The model under review builds one solid part; all positions refer to its coordinate system, in mm. Coordinates: 2 decimals unless noted, no trailing zeros. Order: outer loops, then holes, each group sorted by start corner. A loop starts at its lowest first (then second) coordinate and runs counter-clockwise, first axis right, second up. Notation, with made-up numbers: M -9,-9.75 L 16,-9.75 A17 ccw 16,4.25 Z; hole C 10.25,71 d3. An arc over 180 degrees is marked long. Answer in a Markdown table with one row per item.
from build123d import *

# Parameters (mm, degrees)
F1_DEPTH = 0.127


with BuildPart() as f1:
    # F0 (on Top) → F1 (new body)
    with BuildSketch(Plane.XY):
        with BuildLine():
            ThreePointArc((0, 1.27), (0.371974, 0.371974), (1.27, 0))
            Line((1.27, 0), (24.13, 0))
            ThreePointArc((24.13, 0), (25.028026, 0.371974), (25.4, 1.27))
            Line((25.4, 1.27), (25.4, 5.08))
            ThreePointArc((25.4, 5.08), (25.028026, 5.978026), (24.13, 6.35))
            Line((24.13, 6.35), (16.191119, 6.35))
            ThreePointArc((16.191119, 6.35), (15.720802, 6.234588), (15.357337, 5.914571))
            ThreePointArc((15.357337, 5.914571), (14.503814, 5.622968), (13.97, 6.35))
            Line((13.97, 6.35), (13.97, 21.59))
            ThreePointArc((13.97, 21.59), (14.341974, 22.488026), (15.24, 22.86))
            Line((15.24, 22.86), (45.72, 22.86))
            ThreePointArc((45.72, 22.86), (46.618026, 22.488026), (46.99, 21.59))
            Line((46.99, 21.59), (46.99, -48.600295))
            ThreePointArc((46.99, -48.600295), (46.819852, -49.235295), (46.355, -49.700148))
            ThreePointArc((46.355, -49.700148), (45.890148, -50.165), (45.72, -50.8))
            Line((45.72, -50.8), (45.72, -53.34))
            ThreePointArc((45.72, -53.34), (46.091974, -54.238026), (46.99, -54.61))
            Line((46.99, -54.61), (49.53, -54.61))
            ThreePointArc((49.53, -54.61), (50.428026, -54.238026), (50.8, -53.34))
            Line((50.8, -53.34), (50.8, -50.8))
            ThreePointArc((50.8, -50.8), (50.629852, -50.165), (50.165, -49.700148))
            ThreePointArc((50.165, -49.700148), (49.700148, -49.235295), (49.53, -48.600295))
            Line((49.53, -48.600295), (49.53, 22.86))
            ThreePointArc((49.53, 22.86), (48.786051, 24.656051), (46.99, 25.4))
            Line((46.99, 25.4), (13.97, 25.4))
            ThreePointArc((13.97, 25.4), (12.173949, 24.656051), (11.43, 22.86))
            Line((11.43, 22.86), (11.43, 6.35))
            ThreePointArc((11.43, 6.35), (10.896186, 5.622968), (10.042663, 5.914571))
            ThreePointArc((10.042663, 5.914571), (9.679198, 6.234588), (9.208881, 6.35))
            Line((9.208881, 6.35), (1.27, 6.35))
            ThreePointArc((1.27, 6.35), (0.371974, 5.978026), (0, 5.08))
            Line((0, 5.08), (0, 1.27))
        make_face()
    extrude(amount=F1_DEPTH)


solid = f1.part
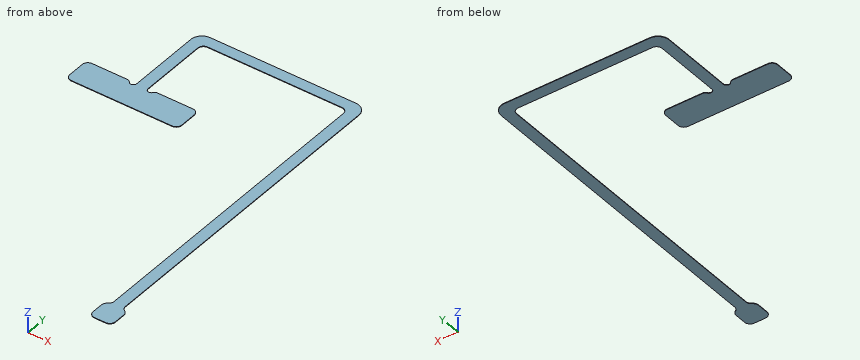
(1) To check wall thickness, follow line 1 (Y direction, x = 27, z = 0.05); line 2 (X direction, y = -35.5, z = 0.05); line 3 (Y direction, x = 47.5, z = 0.05). State the ranges of each line that lie inside material, in increasing order. Write a range as [from, to].
Report:
| item | result |
|---|---|
| line 1 | [22.86, 25.4] |
| line 2 | [46.99, 49.53] |
| line 3 | [-54.61, 25.35] |
(2) Take a section at C-C (y = -9.5). Write out the cut boundary in (x, z), then the cut area to 3 significant figures.
Report:
| item | result |
|---|---|
| outline | M 46.99,0 L 49.53,0 L 49.53,0.13 L 46.99,0.13 Z |
| area | 0.323 mm^2 |
(3) Take a section at D-D (x = 30). Write out the cut boundary in (y, z).
Report:
| item | result |
|---|---|
| outline | M 22.86,0 L 25.4,0 L 25.4,0.13 L 22.86,0.13 Z |
(4) Take a section at A-A (y = 20.5). Write out the cut boundary in (x, z), then the cut area to 3 significant figures.
Report:
| item | result |
|---|---|
| outline | M 11.43,0 L 13.97,0 L 13.97,0.13 L 11.43,0.13 Z; M 46.99,0 L 49.53,0 L 49.53,0.13 L 46.99,0.13 Z |
| area | 0.645 mm^2 |
